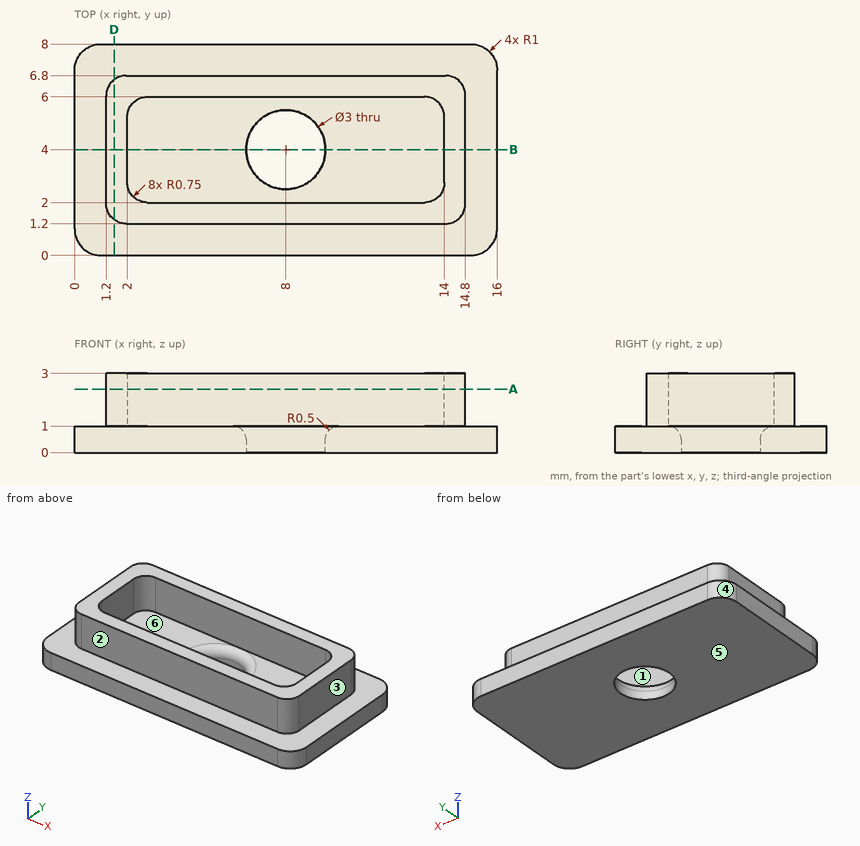
Drawing for the job (mm, zero at the part's lowest x, y, z). A direction names the side the tool comes from. Round coordinates to 2 decimals unless told otherwise and drop trailing zeros. Loops run counter-clockwise (first coordinate to the right, second up) from the corner with the lowest first, then second, coordinate; pieces in that order, holes last. Notation, with made-up numbers: (14.25, 49.25) -> (60.25, 49.25) arc R24 ccw to (60.25, 60.25) -> close; hole circle Ø2 at (-25, 53.5). An arc over 180 degrees is marked (long way). Use one line per item in the form item = value. Start each with the question number.
Item 1: Tool access for the marked faces 1, 2 and 3: list every direction of +Z, -Z, +X, -X, +Y, -Y with a clear straight run to the whole face (end or side of a thin tool).
Item 2: Two-plate mould, pull along X, no slides. Class the marked faces 4, 5 and 6: released by +X, released by -X, zero draft, split by the parting line, or undercut.
Item 3: Band-saw the part on A-A (z = 2.4). List the corners of the cut face in (x, y), plus the area to 3 significant figures.
Item 4: Drill centre lines: line 1 along X through (y, z) = (4, 0.4); line 2 along Y through (x, z) = (8, 0.35); line 3 along Y through (x, z) = (12, 1.75). Where is each one in solid material? Low to high.
Item 5: Band-saw the part on D-D (x = 1.5). List the corners of the cut face in (y, z), plus the area to 3 significant figures.
Item 6: Drop flat-ended pins along their axis: pin 1 Ø0.6 at (x, z) = (9.5, 2.5) entering from +Y; pin 2 Ø0.6 at (y, z) = (4.5, 2.5) entering from +X; pin 3 Ø1 at (y, z) = (2.5, 2.5) entering from -X; pin 4 Ø2.5 at (x, y) = (8, 4) entering from +Z. Give the stop position or say it passes through.
Item 7: Band-saw the part on B-B (y = 4). List the corners of the cut face in (x, z), plus the area to 3 significant figures.
Data:
q1.face_1 = +Z
q1.face_2 = +Z, +X, -X, -Y
q1.face_3 = +Z, +X, +Y, -Y
q2.face_4 = released by -X
q2.face_5 = zero draft
q2.face_6 = undercut
q3.outline = (1.2, 1.95) arc R0.75 ccw to (1.95, 1.2) -> (14.05, 1.2) arc R0.75 ccw to (14.8, 1.95) -> (14.8, 6.05) arc R0.75 ccw to (14.05, 6.8) -> (1.95, 6.8) arc R0.75 ccw to (1.2, 6.05) -> close; hole (2, 2.75) arc R0.75 ccw to (2.75, 2) -> (13.25, 2) arc R0.75 ccw to (14, 2.75) -> (14, 5.25) arc R0.75 ccw to (13.25, 6) -> (2.75, 6) arc R0.75 ccw to (2, 5.25) -> close
q3.area = 28.2 mm^2
q4.line_1 = 0 to 6.5, 9.5 to 16
q4.line_2 = 0 to 2.5, 5.5 to 8
q4.line_3 = 1.2 to 2, 6 to 6.8
q5.outline = (0, 0) -> (8, 0) -> (8, 1) -> (6.65, 1) -> (6.65, 3) -> (1.35, 3) -> (1.35, 1) -> (0, 1) -> close
q5.area = 18.6 mm^2
q6.pin_1 = 6.8
q6.pin_2 = 14.8
q6.pin_3 = 1.2
q6.pin_4 = through
q7.outline = (0, 0) -> (6.5, 0) -> (6.5, 0.5) arc R0.5 ccw to (6, 1) -> (2, 1) -> (2, 3) -> (1.2, 3) -> (1.2, 1) -> (0, 1) -> close; (9.5, 0) -> (16, 0) -> (16, 1) -> (14.8, 1) -> (14.8, 3) -> (14, 3) -> (14, 1) -> (10, 1) arc R0.5 ccw to (9.5, 0.5) -> close
q7.area = 16.1 mm^2
